The listing builds one solid part. Answer for the finished solid, in the listing's coordinates (mm). Round coordinates to 2 decimals unless told otherwise and drop trailing zeros. Order: outer loops, then holes, each group sorted by start corner. A loop starts at its lowest first (then second) coordinate and runs counter-clockwise, first axis right, second up. Notation, with made-up numbers: M 35.5,72.25 L 55.5,72.25 A21 cw 55.5,102.25 Z; hole C -14,34.25 d1. An arc over 180 degrees is marked long. Write item = value, one per line. Start each with the question number.
(1) For a pull along X with two mould halves and no side action, classify faces 1 (the face through (23.846, 7.509, 271.244)), 2 (the face through (-9.76, -0.42, -2.17)), 3 (the face through (0, 0, 525)) as released by +X, released by -X, zero draft, split by the parting line, or undercut.
(2) Straight lines are drawn through the part: probe 1 along X at (y, z) = (-9, 0); probe 2 along Z at (x, y) = (3, 16); probe 3 along Z at (x, y) = (6, 5.5). For each, find the intervals that lie inside material, in ascending order. Write a range as from..to.
(3) Each of these flat-tipped pins is pushed along its axis until it touches: pin 1 (2 mm diameter, centred on y = 11, z = 405.5, fed in from +X); pin 2 (1.5 mm diameter, centred on x = 13, y = -15, fed in from -Z); pin 3 (12 mm diameter, centred on x = 12.5, z = 236.5, fed in from +Y). Where does it stop, or does it pass through?
(4) A cutting plane is placed at A-A, the plane z = 0. Determine the outline of the cut face in (x, y), and give its area (3 significant figures).
(5) A cutting plane is placed at D-D, the plane z = 482. Determine the outline of the cut face in (x, y), and give its area (3 significant figures).
(6) A cutting plane is placed at C-C, the plane y = 7.5. Determine the outline of the cut face in (x, z).
(7) A cutting plane is placed at B-B, the plane x = 0. Determine the outline of the cut face in (y, z), and give its area (3 significant figures).
from build123d import *

# Parameters (mm, degrees)
SKETCH1_R               = 25
BOSS_EXTRUDE1_DEPTH     = 525
SKETCH2_R               = 35
SKETCH2_R_2             = 10
BOSS_EXTRUDE2_DEPTH     = 30
CUT_EXTRUDE1_DEPTH      = 528.019923834
CUT_EXTRUDE1_DEPTH_BACK = 528.019923834
SKETCH2_2_R             = 10


with BuildPart() as part:
    # Sketch1 → Boss-Extrude1 (new body)
    with BuildSketch(Plane.XY):
        Circle(SKETCH1_R)
    extrude(amount=BOSS_EXTRUDE1_DEPTH)

    # Sketch2 → Boss-Extrude2 (add, symmetric)
    with BuildSketch(Plane(origin=(0, 0, 0), x_dir=(1, 0, 0), z_dir=(0, 1, 0))):
        with Locations(Location((0, 0, 0), (0, 0, 270))):
            Circle(SKETCH2_R)
        with Locations(Location((0, 0, 0), (0, 0, 270))):
            Circle(SKETCH2_R_2, mode=Mode.SUBTRACT)
    extrude(amount=BOSS_EXTRUDE2_DEPTH, both=True)

    # Sketch2_2 → Cut-Extrude1 (cut, two sides: drawn at the far end of the back side and taken through both)
    with BuildSketch(Plane(origin=(0, 0, 0), x_dir=(1, 0, 0), z_dir=(0, 1, 0)).offset(-CUT_EXTRUDE1_DEPTH_BACK)):
        with Locations(Location((0, 0, 0), (0, 0, 270))):
            Circle(SKETCH2_2_R)
    extrude(amount=CUT_EXTRUDE1_DEPTH + CUT_EXTRUDE1_DEPTH_BACK, mode=Mode.SUBTRACT)


solid = part.part
Reported:
q1.face_1 = split by the parting line
q1.face_2 = undercut
q1.face_3 = zero draft
q2.probe_1 = -35..-10, 10..35
q2.probe_2 = -34.87..-9.54, 9.54..525
q2.probe_3 = -34.48..-8, 8..525
q3.pin_1 = 22.91
q3.pin_2 = -32.79
q3.pin_3 = 24.14
q4.outline = M -35,-30 L -10,-30 L -10,30 L -35,30 Z; M 10,-30 L 35,-30 L 35,30 L 10,30 Z
q4.area = 3,000 mm²
q5.outline = C 0,0 d50
q5.area = 1,960 mm²
q6.outline = M -23.85,25.62 A35 ccw long 23.85,25.62 L 23.85,525 L -23.85,525 Z; hole C 0,0 d20
q7.outline = M -30,-35 L 30,-35 L 30,-10 L -30,-10 Z; M -30,10 L 30,10 L 30,35 L 25,35 L 25,525 L -25,525 L -25,35 L -30,35 Z
q7.area = 27,500 mm²
